Geometry: final body of the model. Coordinates: model frame, mm. Face numbers are marked on the shaded views. Give positions to 0.01 mm unless a question says otherwise; leave off trailing zeros. Write each loop counter-clockwise with the first axis right and the second up, starting at its lowest first coordinate (ties: lowest second). Pieces come first, ordered by that corner, then holes. Notation, with made-up numbers: (85, -30.5) -> (132, -30.5) arc R18 ccw to (132, -10.5) -> close; hole circle Ø10 at (61.5, 4). An arc over 180 degrees is marked (long way). Answer as a JSON object with one key per item and string values. Group by question number.
(1) Section query B-B on x = 0. Output: boundary loops of the cut face in (y, z).
(2) Contact query for flat-ended pins moving along their axis: pin 1 Ø10 at (y, z) = (39.5, 12.5) entering from +X; pin 2 Ø12 at (x, y) = (6.5, 58) entering from -Z; pin 3 Ø3 at (x, y) = (2, 52) entering from +Z; pin 4 Ø10 at (y, z) = (23.5, 2.5) entering from -X. Output: stop coordinate, or through.
(3) Section query C-C on y = 67.5. Output: boundary loops of the cut face in (x, z), plus the area to 3 significant figures.
(4) Section query A-A on z = 0. Output: boundary loops of the cut face in (x, y).
(5) Material intervals for probe 1 along X at (y, z) = (46.5, 0); probe 2 along Y at (x, z) = (-11.5, 9); probe 3 along Y at (x, z) = (-20.5, 12), sorted ascending.
(6) Draft query along Z for the marked faces 1 and 2. Return one class per face: +Z half, -Z half, draft (parallel to the pull), parting line (faces both ways), or undercut.
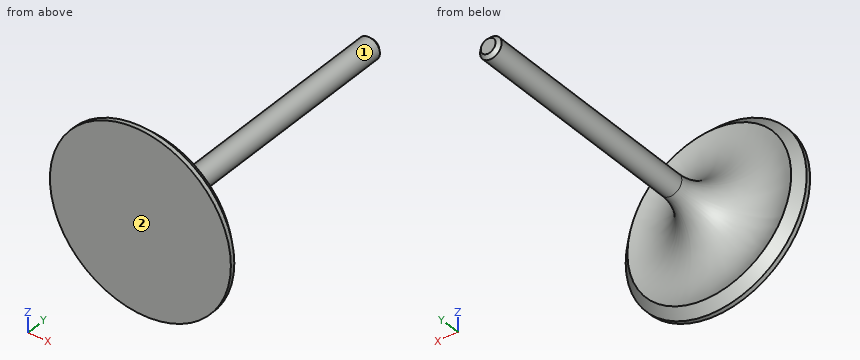
from build123d import *

# Parameters (mm, degrees)
CHAMFER1_SIZE = 1


with BuildPart() as part:
    # Sketch1 → Revolve1 (revolve)
    with BuildSketch(Plane.XY):
        with BuildLine():
            Line((0, 0), (0, 85.55))
            Line((0, 85.55), (3.18, 85.55))
            Line((3.18, 85.55), (3.18, 17.954698654))
            ThreePointArc((3.18, 17.954698654), (9.896609701, 5.315721242), (24.13, 3.81))
            Line((24.13, 3.81), (26.67, 1.27))
            Line((26.67, 1.27), (26.67, 0))
            Line((26.67, 0), (0, 0))
        make_face()
    revolve(axis=Axis((0, 0, 0), (0, 1, 0)))

    # Chamfer1
    chamfer1_edges = [part.edges().sort_by_distance(p)[0] for p in [
        (-3.18, 85.55, 0),
    ]]
    chamfer(chamfer1_edges, length=CHAMFER1_SIZE)


solid = part.part
Answer list:
{
 "1": {"outline": "(0, -26.67) -> (1.27, -26.67) -> (3.81, -24.13) arc R15.25 cw to (17.95, -3.18) -> (84.55, -3.18) -> (85.55, -2.18) -> (85.55, 2.18) -> (84.55, 3.18) -> (17.95, 3.18) arc R15.25 cw to (3.81, 24.13) -> (1.27, 26.67) -> (0, 26.67) -> close"},
 "2": {"pin 1": "through", "pin 2": "z = -3.14", "pin 3": "z = 3.14", "pin 4": "x = -3.18"},
 "3": {"outline": "circle Ø6.36 at (0, 0)", "area": "31.8 mm2"},
 "4": {"outline": "(-26.67, 0) -> (26.67, 0) -> (26.67, 1.27) -> (24.13, 3.81) arc R15.25 cw to (3.18, 17.95) -> (3.18, 84.55) -> (2.18, 85.55) -> (-2.18, 85.55) -> (-3.18, 84.55) -> (-3.18, 17.95) arc R15.25 cw to (-24.13, 3.81) -> (-26.67, 1.27) -> close"},
 "5": {"probe 1": "-3.18 to 3.18", "probe 2": "0 to 3.19", "probe 3": "0 to 3.66"},
 "6": {"face 1": "parting line", "face 2": "draft"}
}
